Model file for the job. Use its own axes, mm. A direction names the side the tool comes from. Round coordinates to 2 decimals unless told otherwise and drop trailing zeros. Order: outer loops, then holes, each group sorted by start corner. A loop starts at its lowest first (then second) coordinate and runs counter-clockwise, first axis right, second up. Notation, with made-up numbers: (31.5, 36.25) -> (43.5, 36.25) arc R29 ccw to (43.5, 62.25) -> close; hole circle Ø8 at (-27.5, -30.5). An arc over 180 degrees is marked (long way). Put each result on its own line as item: value. Start each with the question number.
Q1. Pull direction Y, two halves, no side cores. Call faces 5 (the face through (-8.1, 17.4, -4.9)), 6 (the face through (-12.465, 22.414, -3.819)), 7 (the face through (-12, 9, -8)): released by +Y, released by -Y, zero draft, split by the parting line, or undercut.
Q2. Cut at C-C, the plane x = -52. List the corners of the cut face in (y, z).
Q3. 3-axis set-ups, long thin cutter, end or side, ignore diameter. For faces 1 (the face through (-8.1, 1, -4.9)), 2 (the face through (-38, -1.564, -2)), 3 (the face through (-38, 9, -5)), 4 (the face through (-39, 19.879, -2)): which of +Z, -Z, +X, -X, +Y, -Y reach the whole face in a straight line?
Q4. Cut at D-D, the plane x = -14. List the corners of the cut face in (y, z), and give its area (3 significant figures).
Q5. Flat gauge pins, fed straight in: P1, Ø3, axis at x = -43.5, z = -2.5, coming from the +Y side; P2, Ø1.5, axis at x = -46, y = 21.5, coming from the +Z side; P3, Ø4, axis at x = -18, z = -6.5, coming from the -Y side. Where does each tip first touch, or does it go through?
Q6. Cut at B-B, the plane y = 12. List the corners of the cut face in (x, z), and give its area (3 significant figures).
Q7. Cut at A-A, the plane x = -6.5. List the corners of the cut face in (y, z).
Q8. Probe L1, parallel to Y at x = -6.5, z = -4; L2, parallel to Z at x = -26.5, y = 4; L3, parallel to Y at x = -7.5, z = -7. List the from-to ranges inside material, lowest first.
from build123d import *

# Parameters (mm, degrees)
SALIENTE_EXTRUIR1_DEPTH = 10
CHAFL_N1_SIZE           = 5
CORTAR_EXTRUIR1_DEPTH   = 38


with BuildPart() as part:
    # Croquis1 → Saliente-Extruir1 (new body)
    with BuildSketch(Plane.XY):
        with BuildLine():
            Line((-5, -7.284781413), (-10, -7.284781413))
            Line((-10, -7.284781413), (-10, -1.56358606))
            Line((-10, -1.56358606), (-61.678046138, -1.56358606))
            Line((-61.678046138, -1.56358606), (-61.678046138, 19.878804647))
            Line((-61.678046138, 19.878804647), (-10, 19.878804647))
            Line((-10, 19.878804647), (-10, 25.6))
            Line((-10, 25.6), (-5, 25.6))
            Line((-5, 25.6), (-5, 17.935581083))
            ThreePointArc((-5, 17.935581083), (-8.1, 17.378804647), (-5, 16.82202821))
            Line((-5, 16.82202821), (-5, 1.493190376))
            ThreePointArc((-5, 1.493190376), (-8.1, 0.93641394), (-5, 0.379637504))
            Line((-5, 0.379637504), (-5, -7.284781413))
        make_face()
    extrude(amount=-SALIENTE_EXTRUIR1_DEPTH)

    # Chaflán1
    chafl_n1_edges = [part.edges().sort_by_distance(p)[0] for p in [
        (-10, -1.56358606, -5),
        (-10, 19.878804647, -5),
    ]]
    chamfer(chafl_n1_edges, length=CHAFL_N1_SIZE)

    # Croquis2 → Cortar-Extruir1 (cut)
    with BuildSketch(Plane(origin=(-7.102128625, -7.284781413, 0), x_dir=(0, 0, -1), z_dir=(0, 1, 0))):
        Polygon((5, 7.897871375), (5, 54.575917513), (10, 54.575917513), (10, 2.897871375), align=None)
    extrude(amount=CORTAR_EXTRUIR1_DEPTH, mode=Mode.SUBTRACT)

    # Redondeo1
    # a fillet whose section is not a circle: 0.6 mm, written as the material it takes off along each edge
    with BuildSketch(Plane(origin=(-5, 17.935581083, 3.626773884), x_dir=(-0.6833782327560586, 0.730064511529773, 0), z_dir=(0, 0, -1)), Plane(origin=(-5, 1.493190376, 3.626773884), x_dir=(-0.6833782327560585, 0.7300645115297733, 0), z_dir=(0, 0, -1))) as redondeo1_piece_1:
        with BuildLine():
            Bezier((1.237169264, 0), (0.382683433, 0.358211533), (1.059111562, 0.991383331), weights=[1, 1.857142857, 1])
            Line((1.059111562, 0.991383331), (0, 0))
            ThreePointArc((0, 0), (0.618584632, 0.124414336), (1.237169264, 0))
        make_face()
    extrude(amount=17.253547769, mode=Mode.SUBTRACT)
    with BuildSketch(Plane(origin=(-5, 16.82202821, 3.626773884), x_dir=(0, -1, 0), z_dir=(0, 0, -1)), Plane(origin=(-5, 0.379637504, 3.626773884), x_dir=(0, -1, 0), z_dir=(0, 0, -1))) as redondeo1_piece_2:
        with BuildLine():
            Bezier((1.450709554, 0), (0.524177558, 0), (0.903213375, 0.845454545), weights=[1, 1.857142857, 1])
            ThreePointArc((0.903213375, 0.845454545), (0.536628736, 0.331896782), (0, 0))
            Line((0, 0), (1.450709554, 0))
        make_face()
    extrude(amount=17.253547769, mode=Mode.SUBTRACT)


solid = part.part
Ans:
1. face 5: undercut
1. face 6: released by +Y
1. face 7: zero draft
2. outline: (-1.56, -5) -> (19.88, -5) -> (19.88, 0) -> (-1.56, 0) -> close
3. face 1: +Z, -Z
3. face 2: +Z, -Z, -X, -Y
3. face 3: -Z, -X, +Y, -Y
3. face 4: +Z, -Z, -X, +Y
4. outline: (-2.56, -6) -> (20.88, -6) -> (20.88, 0) -> (-2.56, 0) -> close
4. area: 141 mm^2
5. P1: stops at y = 19.88
5. P2: passes through
5. P3: stops at y = -1.56
6. outline: (-61.68, -5) -> (-15, -5) -> (-10, -10) -> (-5, -10) -> (-5, 0) -> (-61.68, 0) -> close
6. area: 321 mm^2
7. outline: (-7.28, -10) -> (-0.66, -10) -> (-0.66, 0) -> (-7.28, 0) -> close; (2.54, -10) -> (15.78, -10) -> (15.78, 0) -> (2.54, 0) -> close; (18.98, -10) -> (25.6, -10) -> (25.6, 0) -> (18.98, 0) -> close
8. L1: y = -7.28 to -0.66, 2.54 to 15.78, 18.98 to 25.6
8. L2: z = -5 to 0
8. L3: y = -7.28 to -0.31, 2.19 to 16.13, 18.63 to 25.6
